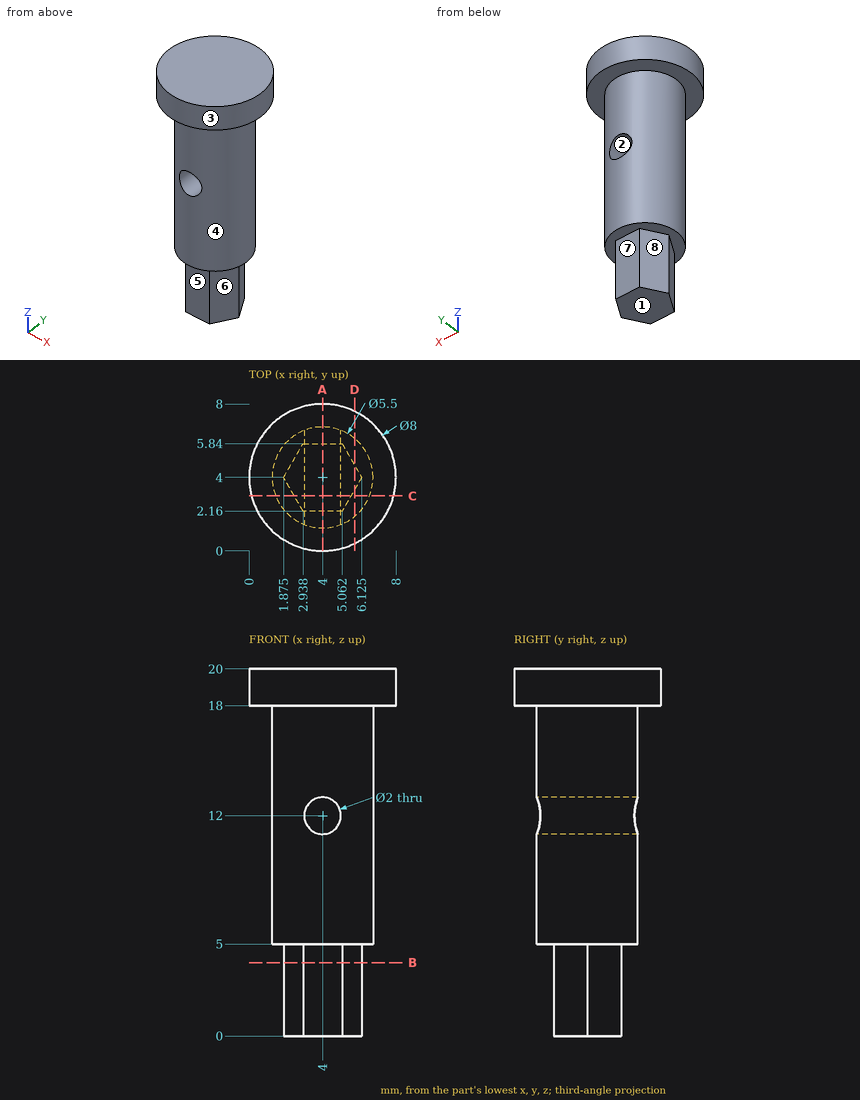
Could you check a few things on this drawing? It's one solid part, dimensions in mm from its lowest x, y, z. A direction names the side the tool comes from. Round coordinates to 2 decimals unless told otherwise and drop trailing zeros. Order: outer loops, then holes, each group sorted by start corner. A loop starts at its lowest first (then second) coordinate and runs counter-clockwise, first axis right, second up. Notation, with made-up numbers: M -39,6 L -19,6 A26 ccw -19,33 Z; hole C -39,11 d7. An arc over 180 degrees is marked long. One line per question, with ' | ' between items.
1) I need wall thicknesses on line 1 (Z direction, x = 4, y = 3.55); line 2 (Z direction, x = 4, y = 0.5); line 3 (X direction, y = 3.75, z = 12). Which ranges of each line are inside material? Lowest first, please.
Checked values:
line 1: z = 0 to 11, 13 to 20 | line 2: z = 18 to 20 | line 3: x = 1.26 to 3, 5 to 6.74
2) We'd pull the mould along X, two halves only. Please class the marked faces 1, 2 and 3: released by +X, released by -X, zero draft, split by the parting line, or undercut.
Checked values:
face 1: zero draft | face 2: undercut | face 3: split by the parting line
3) Imagine slicing it at D-D, the plane x = 5.75. Write out the boundary of the cut face in (y, z).
Checked values:
outline: M 0.4,18 L 1.88,18 L 1.88,5 L 3.35,5 L 3.35,0 L 4.65,0 L 4.65,5 L 6.12,5 L 6.12,18 L 7.6,18 L 7.6,20 L 0.4,20 Z
4) Imagine slicing it at A-A, the plane x = 4. Write out the boundary of the cut face in (y, z).
Checked values:
outline: M 0,18 L 1.25,18 L 1.25,13 L 6.75,13 L 6.75,18 L 8,18 L 8,20 L 0,20 Z; M 1.25,5 L 2.16,5 L 2.16,0 L 5.84,0 L 5.84,5 L 6.75,5 L 6.75,11 L 1.25,11 Z
5) Imagine slicing it at B-B, the plane z = 4. Write out the boundary of the cut face in (x, y) (1 decimal), plus the area to 3 significant figures.
Checked values:
outline: M 1.9,4 L 2.9,2.2 L 5.1,2.2 L 6.1,4 L 5.1,5.8 L 2.9,5.8 Z | area: 11.7 mm²
6) Imagine slicing it at C-C, the plane y = 3. Write out the boundary of the cut face in (x, z).
Checked values:
outline: M 0.13,18 L 1.44,18 L 1.44,5 L 2.45,5 L 2.45,0 L 5.55,0 L 5.55,5 L 6.56,5 L 6.56,18 L 7.87,18 L 7.87,20 L 0.13,20 Z; hole C 4,12 d2
7) I'm going to push flat-ended pins straight in: pin 1 Ø1.7 at (x, z) = (3.5, 2) entering from -Y; pin 2 Ø4 at (x, z) = (5, 10) entering from -Y; pin 3 Ø1.1 at (x, z) = (4, 3) entering from +Y. Where does each tip first touch, or does it pass through?
Checked values:
pin 1: stops at y = 2.16 | pin 2: stops at y = 1.25 | pin 3: stops at y = 5.84
8) On a 3-axis mill with a long thin cutter (end or side, diameter ignored), from which of +Z, -Z, +X, -X, +Y, -Y can I reach the whole of each face in a straight line? I mean the marked faces 4, 5, 6, 7 and 8. Say none if no direction works.
Checked values:
face 4: -Z | face 5: -Z, +X, -X, -Y | face 6: -Z, +X, -Y | face 7: -Z, +X, -X, +Y | face 8: -Z, -X, +Y
